Geometry check sheet. Reference: the model listing, model coordinates, mm. A direction names the side the tool comes from. Round coordinates to 2 decimals unless told otherwise and drop trailing zeros. Order: outer loops, then holes, each group sorted by start corner. A loop starts at its lowest first (then second) coordinate and runs counter-clockwise, first axis right, second up.
(1) Go/stop test with flat-tipped pins: pin 1 (1.6 mm diameter, centred on y = 13, z = 6.5, fed in from -X); pin 2 (1.5 mm diameter, centred on x = -2, y = 1.5, fed in from -Z) (3 decimals); pin 3 (3 mm diameter, centred on y = 4, z = 6.5, fed in from -X); pin 4 (4 mm diameter, centred on x = -12.5, z = 8.5, fed in from +Y). Record where each tip stops, or that it passes through.
(2) Release check for a two-part mould opening along Z. For faces 1 (the face through (-12.5, -0.7, 5)), 2 (the face through (-20, -1, 7)), 3 (the face through (-30, -1, 5)), 4 (the face through (-10, -1, 0)) record: +Z half, -Z half, draft (parallel to the pull), parting line (faces both ways), or undercut.
(3) Sectioned sample at A-A (x = -5). Record the boundary of the cut face in (y, z).
(4) Sectioned sample at B-B (z = 5). Record the boundary of the cut face in (x, y), plus the area to 3 significant figures.
(5) Set-up check for faces 5 (the face through (-10, 13, 5)), 6 (the face through (-21, -1, 3)), 7 (the face through (-4.73, 12.74, 6.22)), 8 (the face through (0, 6, 5)): record each of +Z, -Z, +X, -X, +Y, -Y from which the full face is reachable in a straight line by a thin tool's end or side.
(6) Sectioned sample at C-C (x = -18.5). Record the boundary of the cut face in (y, z).
(7) Material ranges on line 1 along Z through (x, y) = (-5, 12.9); line 2 along Y through (x, z) = (-2.5, 1); line 3 along X through (y, z) = (7, 1), recorded low to high.
(8) Sectioned sample at D-D (z = 1). Record the boundary of the cut face in (x, y).
from build123d import *

# Parameters (mm, degrees)
SM_BASE_FLANGE_1_DEPTH = 10
HOLE_WIZARD_M3_1_D     = 2.5
HOLE_WIZARD_M3_1_DEPTH = 1.5
F_4_0MM_1_D            = 4
CUT_EXTRUDE_1_DEPTH    = 10


# Sheet-metal steps are written as plain solids
with BuildPart() as part:
    # Sketch 1 → 基材-凸緣1 (new body)
    with BuildSketch(Plane.XY):
        with BuildLine():
            Line((-30, 0), (-0.7366, 0))
            ThreePointArc((-0.7366, 0), (-0.215745145, 0.215745145), (0, 0.7366))
            Line((0, 0.7366), (0, 11.2634))
            ThreePointArc((0, 11.2634), (-0.215745145, 11.784254855), (-0.7366, 12))
            Line((-0.7366, 12), (-10, 12))
            Line((-10, 12), (-10, 13.5))
            Line((-10, 13.5), (-0.7366, 13.5))
            ThreePointArc((-0.7366, 13.5), (0.844915027, 12.844915027), (1.5, 11.2634))
            Line((1.5, 11.2634), (1.5, 0.7366))
            ThreePointArc((1.5, 0.7366), (0.844915027, -0.844915027), (-0.7366, -1.5))
            Line((-0.7366, -1.5), (-30, -1.5))
            Line((-30, -1.5), (-30, 0))
        make_face()
    extrude(amount=SM_BASE_FLANGE_1_DEPTH)

    # M3 螺紋孔1
    with Locations(Plane(origin=(0, 13.5, 0), x_dir=(1, 0, 0), z_dir=(0, 1, 0))):
        with Locations((-5, -5)):
            Hole(HOLE_WIZARD_M3_1_D / 2, depth=HOLE_WIZARD_M3_1_DEPTH)

    # Ø4.0mm 定位孔1 (through all)
    with Locations(Plane(origin=(0, -1.5, 0), x_dir=(-1, 0, 0), z_dir=(0, -1, 0))):
        with Locations((26, -5), (18, -5)):
            Hole(F_4_0MM_1_D / 2)

    # 草圖11 → 除料-伸長1 (cut)
    with BuildSketch(Plane(origin=(0, 0, 0), x_dir=(1, 0, 0), z_dir=(0, 1, 0))):
        with BuildLine():
            Line((-14.5, -7), (-26.5, -7))
            ThreePointArc((-26.5, -7), (-28.5, -5), (-26.5, -3))
            Line((-26.5, -3), (-14.5, -3))
            ThreePointArc((-14.5, -3), (-12.5, -5), (-14.5, -7))
        make_face()
    extrude(amount=-CUT_EXTRUDE_1_DEPTH, mode=Mode.SUBTRACT)


solid = part.part
Answer below:
1. pin 1: stops at x = -10
1. pin 2: passes through
1. pin 3: stops at x = 0
1. pin 4: stops at y = 0
2. face 1: undercut
2. face 2: undercut
2. face 3: draft
2. face 4: -Z half
3. outline: (-1.5, 0) - (0, 0) - (0, 10) - (-1.5, 10) - close; (12, 0) - (13.5, 0) - (13.5, 3.75) - (12, 3.75) - close; (12, 6.25) - (13.5, 6.25) - (13.5, 10) - (12, 10) - close
4. outline: (-30, -1.5) - (-28.5, -1.5) - (-28.5, 0) - (-30, 0) - close; (-12.5, -1.5) - (-0.74, -1.5) arc R2.24 ccw to (1.5, 0.74) - (1.5, 11.26) arc R2.24 ccw to (-0.74, 13.5) - (-3.75, 13.5) - (-3.75, 12) - (-0.74, 12) arc R0.74 cw to (0, 11.26) - (0, 0.74) arc R0.74 cw to (-0.74, 0) - (-12.5, 0) - close; (-10, 12) - (-6.25, 12) - (-6.25, 13.5) - (-10, 13.5) - close
4. area: 52.8 mm2
5. face 5: +Z, -Z, -X, +Y
5. face 6: +Y, -Y
5. face 7: +Y
5. face 8: +Z, -Z, -X
6. outline: (-1.5, 0) - (0, 0) - (0, 3) - (-1.5, 3) - close; (-1.5, 7) - (0, 7) - (0, 10) - (-1.5, 10) - close
7. line 1: z = 0 to 3.75, 6.25 to 10
7. line 2: y = -1.5 to 0, 12 to 13.5
7. line 3: x = 0 to 1.5
8. outline: (-30, -1.5) - (-0.74, -1.5) arc R2.24 ccw to (1.5, 0.74) - (1.5, 11.26) arc R2.24 ccw to (-0.74, 13.5) - (-10, 13.5) - (-10, 12) - (-0.74, 12) arc R0.74 cw to (0, 11.26) - (0, 0.74) arc R0.74 cw to (-0.74, 0) - (-30, 0) - close
